The model under review builds one solid part; all positions refer to its coordinate system, in mm. Face numbers are marked on the shaded views. A direction names the side the tool comes from. Coordinates: 2 decimals unless noted, no trailing zeros. Loops run counter-clockwise (first coordinate to the right, second up) from the corner with the lowest first, then second, coordinate; pieces in that order, holes last. Notation, with made-up numbers: (-7.75, 32.5) - (3.25, 32.5) arc R18 cw to (3.25, 53.5) - close; hole circle Ø2 at (23.5, 44.25). An arc over 180 degrees is marked (long way). Use a Markdown table: item, result. Add a question column.
1) Add section D-D, the plane x = 30.5. Give the boundary of the cut face in (y, z), and give its area (3 significant figures).
2) Add section B-B, the plane z = 0.5. Give the boundary of the cut face in (x, y) (1 decimal).
3) Add section C-C, the plane z = -1.5. Give the boundary of the cut face in (x, y).
4) Add section A-A, the plane y = 0. Give the boundary of the cut face in (x, z), and give its area (3 significant figures).
5) To check wall thickness, follow L1, parallel to Z at x = 39, y = 2.75; L2, parallel to Y at x = 1.5, z = -2.5; L3, parallel to X at y = -2, z = -5.5. State the ranges of each line that lie inside material, in increasing order. Write a range as [from, to].
6) Clearance check with flat-ended pins moving along their axes: pin 1 (5 mm diameter, centred on x = 12.5, y = -2, fed in from -Z); pin 2 (5 mm diameter, centred on y = 0, z = -3, fed in from -X). State where each tip first meets the part, or that it passes through.
7) For the marked faces 1 and 2, list the 3-axis set-ups (+Z, -Z, +X, -X, +Y, -Y) from which the entire face can be reached by the end or side of a thin tool; tool diameter is ignored.
```python
from build123d import *

# Parameters (mm, degrees)
F0_R     = 2.778125
F1_DEPTH = 1.984375
F2_DEPTH = 7.9375
F3_D     = 4.7625
F3_DEPTH = 12.7


with BuildPart() as f1:
    # F0 (on Top) → F1 (new body)
    with BuildSketch(Plane.XY):
        with BuildLine():
            Line((41.275, 4.7625), (0, 4.7625))
            ThreePointArc((0, 4.7625), (-4.7625, 0), (0, -4.7625))
            Line((0, -4.7625), (41.275, -4.7625))
            ThreePointArc((41.275, -4.7625), (46.0375, 0), (41.275, 4.7625))
        make_face()
        Circle(F0_R, mode=Mode.SUBTRACT)
        Circle(F0_R)
    extrude(amount=F1_DEPTH)

    # F0 (on Top) → F2 (join)
    with BuildSketch(Plane.XY):
        Circle(F0_R)
    extrude(amount=-F2_DEPTH)

    # F3
    with Locations(Plane(origin=(0, 0, 0), x_dir=(1, 0, 0), z_dir=(0, 0, -1))):
        with Locations((22.225, 0), (41.275, 0)):
            Hole(F3_D / 2, depth=F3_DEPTH)


solid = f1.part
```
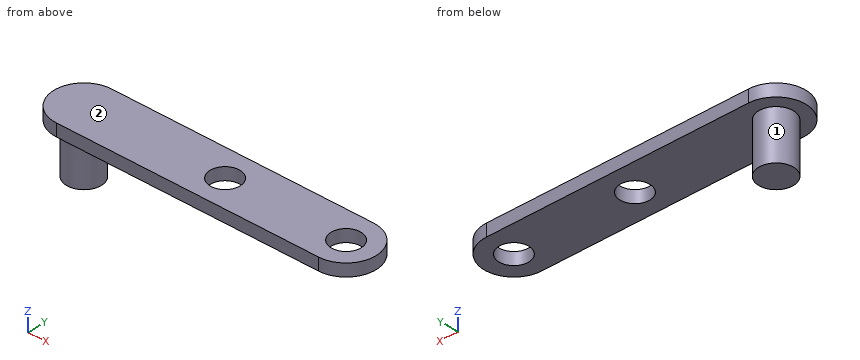
From the geometry:
| question | item | result |
|---|---|---|
| 1 | outline | (-4.76, 0) - (4.76, 0) - (4.76, 1.98) - (-4.76, 1.98) - close |
| 1 | area | 18.9 mm^2 |
| 2 | outline | (0, -4.8) - (41.3, -4.8) arc R4.8 ccw to (41.3, 4.8) - (0, 4.8) arc R4.8 ccw to start; hole circle Ø4.8 at (22.2, 0); hole circle Ø4.8 at (41.3, 0) |
| 3 | outline | circle Ø5.56 at (0, 0) |
| 4 | outline | (-4.76, 0) - (-2.78, 0) - (-2.78, -7.94) - (2.78, -7.94) - (2.78, 0) - (19.84, 0) - (19.84, 1.98) - (-4.76, 1.98) - close; (24.61, 0) - (38.89, 0) - (38.89, 1.98) - (24.61, 1.98) - close; (43.66, 0) - (46.04, 0) - (46.04, 1.98) - (43.66, 1.98) - close |
| 4 | area | 126 mm^2 |
| 5 | L1 | z = [0, 1.98] |
| 5 | L2 | y = [-2.34, 2.34] |
| 5 | L3 | x = [-1.93, 1.93] |
| 6 | pin 1 | stops at z = 0 |
| 6 | pin 2 | stops at x = -2.78 |
| 7 | face 1 | -Z |
| 7 | face 2 | +Z, +X, -X, +Y, -Y |
